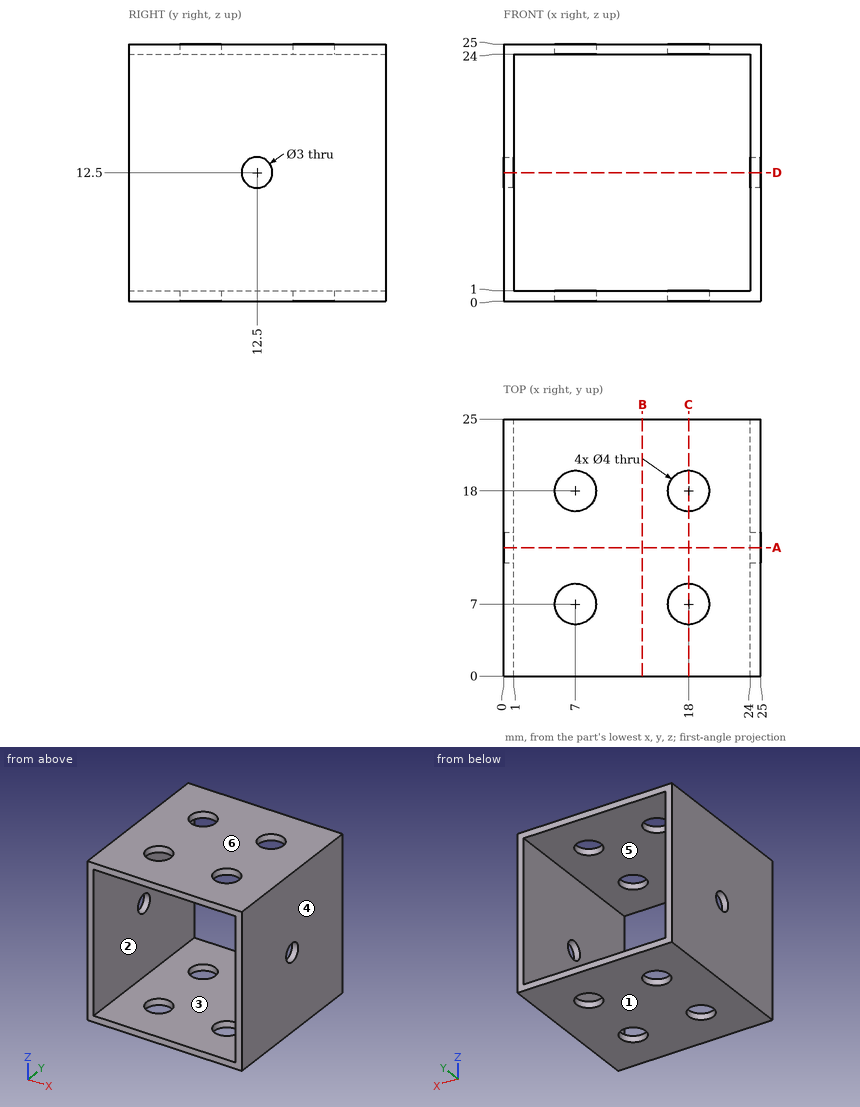
Drawing for the job (mm, zero at the part's lowest x, y, z). A direction names the side the tool comes from. Round coordinates to 2 decimals unless told otherwise and drop trailing zeros. Loops run counter-clockwise (first coordinate to the right, second up) from the corner with the lowest first, then second, coordinate; pieces in that order, holes last. Notation, with made-up numbers: M 38,7 L 49,7 A30 cw 49,45 Z; hole C -22.5,12.25 d5. An arc over 180 degrees is marked long. Use a Markdown table: item, result. Add a question column.
(1) Pull direction Z, two halves, no side cores. Call the marked faces 3, 4, 5 and 6: +Z half, -Z half, draft (parallel to the pull), parting line (faces both ways), or undercut.
(2) Drill centre lines: line 1 (Y direction, x = 18, z = 24.65); line 2 (X direction, y = 13.25, z = 15.75). Where is each one in solid material? Low to high.
(3) Which spindle directions (+Z, -Z, +X, -X, +Y, -Y) get a long thin tool onto all of the face, cutting with end or side? Do the marked faces 1 and 2. Say none if no direction does.
(4) Cut at D-D (z = 12.5). Give the cut face in (x, y).
(5) Cut at A-A (y = 12.5). Give the cut face in (x, z), and give its area (3 significant figures).
(6) Cut at C-C (x = 18). Give the cut face in (y, z).
(7) Cut at B-B (x = 13.5). Give the cut face in (y, z).
Geometry says:
| question | item | result |
|---|---|---|
| 1 | face 3 | undercut |
| 1 | face 4 | draft |
| 1 | face 5 | undercut |
| 1 | face 6 | +Z half |
| 2 | line 1 | y = 0 to 5, 9 to 16, 20 to 25 |
| 2 | line 2 | x = 0 to 1, 24 to 25 |
| 3 | face 1 | -Z, +X, -X, +Y, -Y |
| 3 | face 2 | +Y, -Y |
| 4 | outline | M 0,0 L 1,0 L 1,11 L 0,11 Z; M 0,14 L 1,14 L 1,25 L 0,25 Z; M 24,0 L 25,0 L 25,11 L 24,11 Z; M 24,14 L 25,14 L 25,25 L 24,25 Z |
| 5 | outline | M 0,0 L 25,0 L 25,11 L 24,11 L 24,1 L 1,1 L 1,11 L 0,11 Z; M 0,14 L 1,14 L 1,24 L 24,24 L 24,14 L 25,14 L 25,25 L 0,25 Z |
| 5 | area | 90.0 mm² |
| 6 | outline | M 0,0 L 5,0 L 5,1 L 0,1 Z; M 0,24 L 5,24 L 5,25 L 0,25 Z; M 9,0 L 16,0 L 16,1 L 9,1 Z; M 9,24 L 16,24 L 16,25 L 9,25 Z; M 20,0 L 25,0 L 25,1 L 20,1 Z; M 20,24 L 25,24 L 25,25 L 20,25 Z |
| 7 | outline | M 0,0 L 25,0 L 25,1 L 0,1 Z; M 0,24 L 25,24 L 25,25 L 0,25 Z |
